Source: CAD feature listing. Evaluate the final solid. Frame: model axes, mm. Face numbers are marked on the shaded views. A direction names the side the tool comes from. Round coordinates to 2 decimals unless told otherwise and drop trailing zeros. Order: outer loops, then holes, each group sorted by start corner. A loop starts at its lowest first (then second) coordinate and runs counter-clockwise, first axis right, second up. Notation, with made-up numbers: (34, 56) - (82, 56) arc R26 cw to (82, 84) - close; hole circle Ø2 at (-26.75, 31.5). An arc over 180 degrees is marked (long way). Use one line per item in the form item = value. Start each with the question number.
Q1. Cut plane B-B, the plane z = -5. Return the cut outline in (x, y).
Q2. Set-up query: the marked faces 1, 2, 3 and 4. Return all of +Z, -Z, +X, -X, +Y, -Y with unobstructed straight access to the full face (end or side cutting, diameter ignored); none if empty.
Q3. Pin query (flat end, axial travel): pin 1 Ø2 at (x, y) = (-23.5, 49.5) entering from -Z; pin 2 Ø11.5 at (y, z) = (-127, 52) entering from +X; pin 3 Ø4 at (x, y) = (-94.5, 48) entering from +Z. Return the tip coordinate at first contact, or that it passes through.
Q4. Ray query, line 1 (Z direction, x = -48, y = 49); line 2 (Y direction, x = -84, z = -10); line 3 (Y direction, x = -90.5, z = -57.5). Return the intervals inside material, ascending. Write a range as [from, to].
Q5. Cut plane A-A, the plane y = 107.5. Return the cut outline in (x, z).
Q6. Cut plane C-C, the plane x = -71. Return the cut outline in (y, z).
Q7. Cut plane D-D, the plane z = 16.5. Return the cut outline in (x, y).
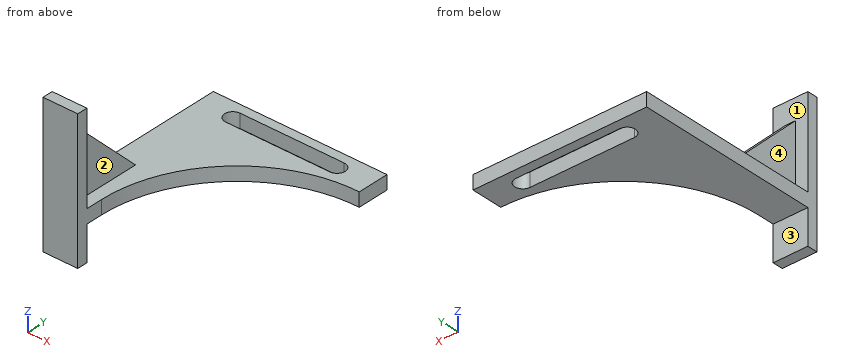
from build123d import *

# Parameters (mm, degrees)
BOSS_EXTRUDE1_DEPTH = 20
CUT_EXTRUDE1_DEPTH  = 80
SKETCH3_W           = 15
SKETCH3_H           = 100
BOSS_EXTRUDE2_DEPTH = 100
SKETCH10_W          = 50
SKETCH10_H          = 200
BOSS_EXTRUDE4_DEPTH = 15
CUT_EXTRUDE3_DEPTH  = 166


with BuildPart() as part:
    # Sketch1 → Boss-Extrude1 (new body)
    with BuildSketch(Plane.XY):
        with BuildLine():
            Line((-75, -132.5), (-125, -132.5))
            Line((-125, -132.5), (-125, 132.5))
            Line((-125, 132.5), (125, 132.5))
            Line((125, 132.5), (125, 86.875222581))
            ThreePointArc((125, 86.875222581), (-16.12613386, 31.381561178), (-75, -108.368215209))
            Line((-75, -108.368215209), (-75, -132.5))
        make_face()
    extrude(amount=-BOSS_EXTRUDE1_DEPTH)

    # Sketch2 → Cut-Extrude1 (cut)
    with BuildSketch(Plane.XY):
        with BuildLine():
            Line((-75, 119.25), (75, 119.25))
            ThreePointArc((75, 119.25), (86.75, 107.5), (75, 95.75))
            Line((75, 95.75), (-75, 95.75))
            ThreePointArc((-75, 95.75), (-86.75, 107.5), (-75, 119.25))
        make_face()
    extrude(amount=-CUT_EXTRUDE1_DEPTH, mode=Mode.SUBTRACT)

    # Sketch3 → Boss-Extrude2 (add)
    with BuildSketch(Plane.XY):
        with Locations((-100, -82.5)):
            Rectangle(SKETCH3_W, SKETCH3_H)
    extrude(amount=BOSS_EXTRUDE2_DEPTH)

    # Sketch10 → Boss-Extrude4 (add)
    with BuildSketch(Plane.XZ.offset(132.5)):
        with Locations((-100, 30)):
            Rectangle(SKETCH10_W, SKETCH10_H)
    extrude(amount=BOSS_EXTRUDE4_DEPTH)

    # Sketch11 → Cut-Extrude3 (cut)
    with BuildSketch(Plane(origin=(-92.5, 0, 0), x_dir=(0, 0, -1), z_dir=(1, 0, 0))):
        Polygon((0, -32.5), (-100, -132.5), (-100, -32.5), align=None)
    extrude(amount=-CUT_EXTRUDE3_DEPTH, mode=Mode.SUBTRACT)


solid = part.part
Completed:
q1.outline = (-125, -147.5) - (-75, -147.5) - (-75, -108.37) arc R195.3 cw to (125, 86.88) - (125, 132.5) - (-125, 132.5) - close; hole (-75, 95.75) - (75, 95.75) arc R11.75 ccw to (75, 119.25) - (-75, 119.25) arc R11.75 ccw to start
q2.face_1 = +Z, +Y
q2.face_2 = +Z, +X, +Y
q2.face_3 = -Z, +X, -X, +Y
q2.face_4 = +Z, -X, +Y
q3.pin_1 = -20
q3.pin_2 = -75
q3.pin_3 = 0
q4.line_1 = [-20, 0]
q4.line_2 = [-147.5, 99.95], [115.05, 132.5]
q4.line_3 = [-147.5, -132.5]
q5.outline = (-125, -20) - (-86.75, -20) - (-86.75, 0) - (-125, 0) - close; (86.75, -20) - (125, -20) - (125, 0) - (86.75, 0) - close
q6.outline = (-69.04, -20) - (95.75, -20) - (95.75, 0) - (-69.04, 0) - close; (119.25, -20) - (132.5, -20) - (132.5, 0) - (119.25, 0) - close
q7.outline = (-125, -147.5) - (-75, -147.5) - (-75, -132.5) - (-92.5, -132.5) - (-92.5, -49) - (-107.5, -49) - (-107.5, -132.5) - (-125, -132.5) - close
